from build123d import *

# Parameters (mm, degrees)
SKETCH3_W                    = 6
SKETCH3_H                    = 50
REVOLVE1_ANGLE               = 23
REVOLVE1_OTHER_WAY_ANGLE     = 23
SKETCH4_W                    = 6
SKETCH4_H                    = 30
CUT_REVOLVE1_ANGLE           = 15
CUT_REVOLVE1_OTHER_WAY_ANGLE = 15
FILLET1_R                    = 6


with BuildPart() as part:
    # Sketch3 → Revolve1 (revolve)
    with BuildSketch(Plane(origin=(0, 0, 0), x_dir=(1, 0, 0), z_dir=(0, 1, 0))):
        with Locations((104.15, 0)):
            Rectangle(SKETCH3_W, SKETCH3_H)
    revolve(axis=Axis((0, 0, 17.71875), (0, 0, -1)), revolution_arc=REVOLVE1_ANGLE)

    # Sketch3 → Revolve1 other way (revolve)
    with BuildSketch(Plane(origin=(0, 0, 0), x_dir=(1, 0, 0), z_dir=(0, 1, 0))):
        with Locations((104.15, 0)):
            Rectangle(SKETCH3_W, SKETCH3_H)
    revolve(axis=Axis((0, 0, 17.71875), (0, 0, 1)), revolution_arc=REVOLVE1_OTHER_WAY_ANGLE)

    # Sketch4 → Cut-Revolve1 (revolve, cut)
    with BuildSketch(Plane(origin=(0, 0, 0), x_dir=(1, 0, 0), z_dir=(0, 1, 0))):
        with Locations((104.15, 0)):
            Rectangle(SKETCH4_W, SKETCH4_H)
    revolve(axis=Axis((0, 0, 15), (0, 0, -1)), revolution_arc=CUT_REVOLVE1_ANGLE, mode=Mode.SUBTRACT)

    # Sketch4 → Cut-Revolve1 other way (revolve, cut)
    with BuildSketch(Plane(origin=(0, 0, 0), x_dir=(1, 0, 0), z_dir=(0, 1, 0))):
        with Locations((104.15, 0)):
            Rectangle(SKETCH4_W, SKETCH4_H)
    revolve(axis=Axis((0, 0, 15), (0, 0, 1)), revolution_arc=CUT_REVOLVE1_OTHER_WAY_ANGLE, mode=Mode.SUBTRACT)

    # Fillet1
    fillet1_edges = [part.edges().sort_by_distance(p)[0] for p in [
        (100.601174808, -26.956003547, 15),
        (100.601174808, -26.956003547, -15),
        (100.601174808, 26.956003547, 15),
        (100.601174808, 26.956003547, -15),
    ]]
    fillet(fillet1_edges, radius=FILLET1_R)


solid = part.part
Geometry check sheet. Reference: the model listing, model coordinates, mm. A direction names the side the tool comes from. Round coordinates to 2 decimals unless told otherwise and drop trailing zeros. Write each loop counter-clockwise with the first axis right and the second up, starting at its lowest first coordinate (ties: lowest second). Pieces come first, ordered by that corner, then holes. Notation, with made-up numbers: (1, 55.25) -> (27, 55.25) arc R30 cw to (27, 94.25) -> close; hole circle Ø3 at (43.25, 67). An arc over 180 degrees is marked (long way). One line per item, written item: value. Start each with the question number.
(1) Cross-section at A-A, the plane z = 3.5. Record the cut outline in (x, y).
(2) Access from +Z, -Z, +X, -X, +Y, -Y to the whole of each face (thin tool, end or side, straight path). Record for faces 1 (the cylindrical face through (101, 25.29, 13.2)), 2 (the cylindrical face through (101.15, -0.57, -17.02)).
(3) Cross-section at C-C, the plane z = -19.5. Record the cut outline in (x, y), and give its area (3 significant figures).
(4) Scan lines: line 1 (Z direction, x = 102.75, y = 11); line 2 (Y direction, x = 99, z = 11.5); line 3 (Y direction, x = 98.5, z = 12.5). Record each from-to range of solid material in increasing order. Write a range as [from, to].
(5) Go/stop test with flat-tipped pins: pin 1 Ø6 at (x, z) = (95.5, 5.5) entering from -Y; pin 2 Ø12 at (y, z) = (33, 6.5) entering from +X. Record where each tip stops, or that it passes through.
(6) Cross-section at B-B, the plane x = 95. Record the cut outline in (y, z).
(7) Draft check along Z on faces 3 (the cylindrical face through (101, -25.29, 13.2)), 4 (the flat face through (102, 1, 25)), 5 (the flat face through (95.832, -40.678, -0.35)). Enter one of: +Z half, -Z half, draft (parallel to the pull), parting line (faces both ways), or undercut.
Answer:
1. outline: (93.11, -39.52) -> (98.63, -41.87) arc R107.15 ccw to (103.5, -27.73) -> (97.7, -26.18) arc R101.15 cw to start; (93.11, 39.52) arc R101.15 cw to (97.7, 26.18) -> (103.5, 27.73) arc R107.15 ccw to (98.63, 41.87) -> close
2. face 1: +X
2. face 2: +Z, -Z, -X
3. outline: (93.11, -39.52) -> (98.63, -41.87) arc R107.15 ccw to (98.63, 41.87) -> (93.11, 39.52) arc R101.15 cw to start
3. area: 502 mm²
4. line 1: [-25, -15], [15, 25]
4. line 2: [-40.99, -25.96], [25.96, 40.99]
4. line 3: [-41.81, -25.23], [25.23, 41.81]
5. pin 1: y = -41.81
5. pin 2: x = 103.5
6. outline: (-40.33, -25) -> (-34.73, -25) -> (-34.73, 25) -> (-40.33, 25) -> close; (34.73, -25) -> (40.33, -25) -> (40.33, 25) -> (34.73, 25) -> close
7. face 3: undercut
7. face 4: +Z half
7. face 5: draft
